Autodesk Inventor part; units mm, degrees
ref_plane "Work Plane1" through (0, -7.1, 18) normal (-1, 0, 0) x (0, 0, 1)
ref_plane "XZ Plane" through (0, 0, 0) normal (0, 1, 0) x (-1, 0, 0)
ref_plane "XY Plane" through (0, 0, 0) normal (0, 0, 1) x (1, 0, 0)
sketch "Sketch1" plane through (0, 0, 0) normal (0, 0, 1) x (1, 0, 0)
  circle A0 centre (0, 0) radius 4.9
  circle A1 centre (0, 0) radius 6.1
  line L0 (-10.1, -7.1) -> (10.1, -7.1)
  line L1 (10.1, -7.1) -> (10.1, 7.1)
  line L2 (10.1, 7.1) -> (-10.1, 7.1)
  line L3 (-10.1, 7.1) -> (-10.1, -7.1)
  line L4 (-10.1, -7.1) -> (10.1, 7.1) construction
  line L5 (10.1, -7.1) -> (-10.1, 7.1) construction
  dimension "d0" = 9.8
  dimension "d1" = 12.2
  dimension "d3" = 4
  dimension "d4" = 1
extrude "Extrusion1" add sketch "Sketch1" along normal blind 18
sketch "Sketch2" plane through (0, 0, 18) normal (0, 0, 1) x (1, 0, 0)
  circle A0 centre (0, 0) radius 4.9
extrude "Extrusion2" add sketch "Sketch2" along normal blind 2
sketch "Sketch3" plane through (0, 0, 0) normal (0, 0, -1) x (-1, 0, 0)
  line L0 (-10.1, -7.1) -> (-10.1, 7.1)
  line L1 (10.1, -7.1) -> (-10.1, -7.1)
  line L2 (10.1, 7.1) -> (10.1, -7.1)
  line L3 (-10.1, 7.1) -> (10.1, 7.1)
  circle A0 centre (0, 0) radius 6.1
extrude "Extrusion3" add sketch "Sketch3" along normal blind 3 contours L0 L3 L2 L1 | A0
ref_plane "Work Plane1" through (0, -7.1, 18) normal (-1, 0, 0) x (0, 0, 1)
sketch "Sketch6" plane through (-10.1, 7.1, 18) normal (0, 1, 0) x (1, 0, 0)
  line L0 (5.2, 18) -> (15, 18)
  line L1 (16.2, 18) -> (4, 18)
  line L2 (20.2, 0) -> (0, 0)
  line L3 (0, 21) -> (20.2, 21)
  line L4 (16.2, 0) -> (16.2, 18)
  line L5 (4, 0) -> (4, 18)
  circle A0 centre (10.1, 10) radius 2.05
  line L6 (0, 21) -> (0, 0)
  line L7 (20.2, 21) -> (20.2, 0)
  point P0 (10.1, 18)
  point P1 (10.1, 18)
  dimension "d49" = 4.1
  dimension "d50" = 10
extrude "Extrusion12" cut sketch "Sketch6" against normal blind 100 contours A0
fillet "Fillet5" radius 2 4 edges at (10.1, 0, 18) (-10.1, 0, 18) (10.1, 0, -3) (-10.1, 0, -3)
sketch "Sketch14" plane through (-8.1, -7.1, -3) normal (0, -1, 0) x (1, 0, 0)
  circle A0 centre (8.1, 11) radius 2.05
  line L0 (8.1, 15.0415) -> (11.6, 13.0207)
  line L1 (11.6, 13.0207) -> (11.6, 8.9793)
  line L2 (11.6, 8.9793) -> (8.1, 6.9585)
  line L3 (8.1, 6.9585) -> (4.6, 8.9793)
  line L4 (4.6, 8.9793) -> (4.6, 13.0207)
  line L5 (4.6, 13.0207) -> (8.1, 15.0415)
  circle A1 centre (8.1, 11) radius 8
  point P0 (8.1, 3)
  dimension "d69" = 7
  dimension "d73" = 16
sketch "Sketch15" plane through (0, -12.1, 8) normal (0, -1, 0) x (1, 0, 0)
  line L0 (3.4, -1) -> (4.8, -1)
  line L1 (4.8, -1) -> (4.8, -7.2415)
  line L2 (4.8, -7.2415) -> (3.4, -7.2415)
  line L3 (3.4, -7.2415) -> (3.4, -1)
  line L4 (3.4, -1) -> (4.8, -7.2415) construction
  line L5 (4.8, -1) -> (3.4, -7.2415) construction
  line L6 (0, 16.6) -> (0, -15.6)
  circle A0 centre (0, 0) radius 2.05
  circle A1 centre (0, 0) radius 4.5
  circle A2 centre (0, 0) radius 8
  line L7 (0, 4.0415) -> (3.5, 2.0207)
  line L8 (3.5, 2.0207) -> (3.5, -2.0207)
  line L9 (3.5, -2.0207) -> (0, -4.0415)
  line L10 (0, -4.0415) -> (-3.5, -2.0207)
  line L11 (-3.5, -2.0207) -> (-3.5, 2.0207)
  line L12 (-3.5, 2.0207) -> (0, 4.0415)
  circle A3 centre (0, 0) radius 8
  line L13 (1.4, -7.8765) -> (3.4, -7.8765)
  line L14 (3.4, -7.8765) -> (3.4, -4.8765)
  line L15 (3.4, -4.8765) -> (1.4, -4.8765)
  line L16 (1.4, -4.8765) -> (1.4, -7.8765)
  line L17 (4.8, -6.4) -> (6.8, -6.4)
  line L18 (6.8, -6.4) -> (6.8, -2.4)
  line L19 (6.8, -2.4) -> (4.8, -2.4)
  line L20 (4.8, -2.4) -> (4.8, -6.4)
  line L21 (4.8, 1) -> (3.4, 1)
  line L22 (3.4, 1) -> (3.4, 7.2415)
  line L23 (3.4, 7.2415) -> (4.8, 7.2415)
  line L24 (4.8, 7.2415) -> (4.8, 1)
  line L25 (4.8, 1) -> (3.4, 7.2415) construction
  line L26 (3.4, 1) -> (4.8, 7.2415) construction
  line L27 (4.8, 6.4) -> (6.8, 6.4)
  line L28 (6.8, 6.4) -> (6.8, 3.4)
  line L29 (6.8, 3.4) -> (4.8, 3.4)
  line L30 (4.8, 3.4) -> (4.8, 6.4)
  line L31 (1.4, 8.7415) -> (3.4, 8.7415)
  line L32 (3.4, 8.7415) -> (3.4, 5.7415)
  line L33 (3.4, 5.7415) -> (1.4, 5.7415)
  line L34 (1.4, 5.7415) -> (1.4, 8.7415)
  point P0 (0, -8)
  point P1 (4.1, -4.1208)
  point P2 (2.05, 0)
  point P3 (4.8, -6.4)
  point P4 (6.8, -4.2143)
  point P5 (4.1, 4.1208)
  point P6 (4.8, 3.4)
  point P7 (6.8, 4.2143)
  point P8 (4.8, 6.4)
  point P9 (1.4, 7.8765)
  point P10 (4.8, 6.4)
  dimension "d74" = 4.1
  dimension "d75" = 1.4
  dimension "d76" = 9
  dimension "d77" = 1
  dimension "d78" = 2
  dimension "d79" = 3
  dimension "d80" = 2
  dimension "d81" = 4
  dimension "d84" = 1.4
  dimension "d85" = 1
  dimension "d86" = 4.1
  dimension "d87" = 2
  dimension "d88" = 3
  dimension "d89" = 2
  dimension "d90" = 3
  dimension "d97" = 1.5
sketch "Sketch16" plane through (-3.5, -7.1, 5.9793) normal (0, -1, 0) x (1, 0, 0)
  line L0 (3.5, 6.0622) -> (0, 4.0415)
  line L1 (0, 4.0415) -> (0, 0)
  line L2 (0, 0) -> (3.5, -2.0207)
  line L3 (3.5, -2.0207) -> (7, 0)
  line L4 (7, 0) -> (7, 4.0415)
  line L5 (7, 4.0415) -> (3.5, 6.0622)
  circle A0 centre (3.5, 2.0207) radius 2.05
  point P0 (3.5, -5.9793)
sketch "Sketch17" plane through (-8.1, -12.1, -3) normal (0, -1, 0) x (1, 0, 0)
  arc A0 (12.9, 17.4) -> (11.5, 18.2415) centre (8.1, 11) ccw
  circle A1 centre (8.1, 11) radius 25
  circle A2 centre (8.1, 11) radius 8
  point P0 (8.1, 3)
  point P1 (9.5, 18.8765)
  point P2 (9.5, 18.8765)
  point P3 (14.9, 15.2143)
  dimension "d94" = 17
sketch "Sketch18" plane through (-8.1, -7.1, -3) normal (0, -1, 0) x (1, 0, 0)
  circle A0 centre (8.1, 11) radius 25
  arc A1 (-2, 2) -> (0, 0) centre (0, 2) ccw
  line L0 (16.2, 0) -> (0, 0)
  arc A2 (16.2, 0) -> (18.2, 2) centre (16.2, 2) ccw
  line L1 (18.2, 19) -> (18.2, 2)
  arc A3 (18.2, 19) -> (16.2, 21) centre (16.2, 19) ccw
  line L2 (0, 21) -> (16.2, 21)
  arc A4 (0, 21) -> (-2, 19) centre (0, 19) ccw
  line L3 (-2, 2) -> (-2, 19)
  circle A5 centre (8.1, 11) radius 8
  point P0 (8.1, 3)
sketch "Sketch20" plane through (0, -12.1, 8) normal (0, -1, 0) x (1, 0, 0)
  circle A0 centre (0, 0) radius 25
  circle A1 centre (0, 0) radius 22
  point P0 (0, -8)
  dimension "d104" = 3
sketch "Sketch21" plane through (-8.1, -5.1, -3) normal (0, 1, 0) x (1, 0, 0)
  arc A0 (11.4466, -35.775) -> (4.7534, -35.775) centre (8.1, -11) ccw
  arc A1 (11.3011, -32.7659) -> (4.8989, -32.7659) centre (8.1, -11) ccw
  circle A2 centre (8.1, -11) radius 2.05
  circle A3 centre (8.1, -11) radius 22
  circle A4 centre (8.1, -11) radius 22
  line L0 (0.1, -31.4939) -> (0.1, -34.6854)
  line L1 (16.1, -31.4939) -> (16.1, -34.6854)
  point P0 (8.1, -3)
  point P1 (11.4466, -33.7552)
  point P2 (4.7534, -33.7552)
  point P3 (16.1, -31.4939)
  point P4 (18.1, -31.7123)
  point P5 (-1.9, -31.7123)
  dimension "d107" = 3
  dimension "d108" = 8
  dimension "d109" = 8
  dimension "d124" = 37
  dimension "d125" = 19
  dimension "d126" = 1.5
  dimension "d127" = 1.5
  dimension "d130" = 360
properties part number "Primary_hinge_V2"
Geometry: final body of the model. Coordinates: model frame, mm. A direction names the side the tool comes from. Round coordinates to 2 decimals unless told otherwise and drop trailing zeros. Write each loop counter-clockwise with the first axis right and the second up, starting at its lowest first coordinate (ties: lowest second). Pieces come first, ordered by that corner, then holes.
Item 1: Section query A-A (z = 1.25). Return loops of the section in (x, y), plus the area to 3 significant figures.
Item 2: Material intervals for L1, parallel to Y at x = 0, z = 13.75; L2, parallel to Y at x = 2.75, z = 6.25; L3, parallel to X at y = -0.75, z = 15.5, sorted ascending.
Item 3: Section query C-C (y = 0). Return loops of the section in (x, z).
Item 4: Section query B-B (x = 0). Return loops of the section in (y, z).
Item 5: Mould query, pull axis Z, two halves, no side actions, for faces 1 (the face through (-9.5, -0.1, 17.43)), 2 (the face through (10.1, 0, 7)), 3 (the face through (1.955, -6.564, 7.384)). Classes: +Z half, -Z half, draft (parallel to the pull), parting line (faces both ways), or undercut.
Item 6: Set-up query: faces 4 (the face through (2, 7.1, 7)), 5 (the face through (5.82, -1.83, 8.87)). Return all of +Z, -Z, +X, -X, +Y, -Y with unobstructed straight access to the full face (end or side cutting, diameter ignored); none if empty.
Item 7: Section query D-D (z = 8). Return loops of the section in (x, y).
Completed:
1. outline: (-10.1, -7.1) - (10.1, -7.1) - (10.1, 7.1) - (-10.1, 7.1) - close; circle Ø9.8 at (0, 0); hole circle Ø12.2 at (0, 0)
1. area: 245 mm2
2. L1: y = -7.1 to -6.1, -4.9 to 4.9, 6.1 to 7.1
2. L2: y = -7.1 to -5.44, -4.06 to 4.06, 5.44 to 7.1
2. L3: x = -10.1 to -6.05, -4.84 to 4.84, 6.05 to 10.1
3. outline: (-10.1, -1) arc R2 ccw to (-8.1, -3) - (8.1, -3) arc R2 ccw to (10.1, -1) - (10.1, 16) arc R2 ccw to (8.1, 18) - (6.1, 18) - (6.1, 0) - (4.9, 0) - (4.9, 20) - (-4.9, 20) - (-4.9, 0) - (-6.1, 0) - (-6.1, 18) - (-8.1, 18) arc R2 ccw to (-10.1, 16) - close; hole circle Ø4.1 at (0, 8)
4. outline: (-7.1, -3) - (7.1, -3) - (7.1, 5.95) - (6.1, 5.95) - (6.1, 0) - (4.9, 0) - (4.9, 5.95) - (-4.9, 5.95) - (-4.9, 0) - (-6.1, 0) - (-6.1, 5.95) - (-7.1, 5.95) - close; (-7.1, 10.05) - (-6.1, 10.05) - (-6.1, 18) - (-7.1, 18) - close; (-4.9, 10.05) - (4.9, 10.05) - (4.9, 20) - (-4.9, 20) - close; (6.1, 10.05) - (7.1, 10.05) - (7.1, 18) - (6.1, 18) - close
5. face 1: +Z half
5. face 2: draft
5. face 3: undercut
6. face 4: +Z, -Z, +X, -X, +Y
6. face 5: +Z
7. outline: (-10.1, -7.1) - (-2.05, -7.1) - (-2.05, -5.75) arc R6.1 cw to (-2.05, 5.75) - (-2.05, 7.1) - (-10.1, 7.1) - close; (-2.05, -4.45) - (-2.05, 4.45) arc R4.9 ccw to start; (2.05, -7.1) - (10.1, -7.1) - (10.1, 7.1) - (2.05, 7.1) - (2.05, 5.75) arc R6.1 cw to (2.05, -5.75) - close; (2.05, -4.45) arc R4.9 ccw to (2.05, 4.45) - close
